Work out the finished part from the listing and answer in its coordinate system (mm). A direction names the side the tool comes from. Round coordinates to 2 decimals unless told otherwise and drop trailing zeros. Loops run counter-clockwise (first coordinate to the right, second up) from the corner with the lowest first, then second, coordinate; pieces in that order, holes last.
from build123d import *

# Parameters (mm, degrees)
ZAOKR_GLENIE2_R  = 2
SFAZOWANIE1_SIZE = 3


with BuildPart() as part:
    # Szkic1 → Obrót1 (revolve)
    with BuildSketch(Plane(origin=(0, 0, 0), x_dir=(1, 0, 0), z_dir=(0, 1, 0))):
        Polygon((15, 65), (-15, 65), (-15, 76), (-7.5, 76), (-7.5, 84), (-15, 84), (-15, 95), (15, 95), (15, 84), (7.5, 84), (7.5, 76), (15, 76), align=None)
    revolve(axis=Axis((0, 0, 0), (-1, 0, 0)))

    # Zaokrąglenie2
    zaokr_glenie2_edges = [part.edges().sort_by_distance(p)[0] for p in [
        (-7.5, 0, 84),
        (7.5, 0, 84),
        (7.5, 0, 76),
    ]]
    fillet(zaokr_glenie2_edges, radius=ZAOKR_GLENIE2_R)

    # Sfazowanie1
    sfazowanie1_edges = [part.edges().sort_by_distance(p)[0] for p in [
        (15, 0, 76),
        (-15, 0, 76),
        (-15, 0, 95),
        (15, 0, 95),
    ]]
    chamfer(sfazowanie1_edges, length=SFAZOWANIE1_SIZE)


solid = part.part
Item 1: Determine the mould class of faces 1 (the face through (7.5, 30, -73)), 2 (the face through (14.854, 89.954, 19.975)), 3 (the face through (15, 43, 49)) for opening direction Y: pulls with the +Y half, pulls with the -Y half, needs draft (parallel to the pull), parting line crosses it, or undercut.
Item 2: Section A-A, the plane x = 1.5 is taken. Give the vertices of the cut face in (y, z), plus the area to 3 significant figures.
Item 3: Straight lines are drawn through the part: line 1 (Y direction, x = -10.85, z = 0); line 2 (Z direction, x = 4.25, y = 0); line 3 (Z direction, x = 13.85, y = 0). For each, find the intervals that lie inside material, in ascending order.
Item 4: Each of these flat-tipped pins is pushed along its axis until it touches: P1, Ø5, axis at x = -1, y = -32, coming from the -Z side; P2, Ø12, axis at x = 6, z = 39, coming from the -Y side; P3, Ø10, axis at x = -5, y = -68, coming from the +Z side. Where does it stop, or does it pass through?
Item 5: For faces 4 (the face through (-9.718, 67.425, -35.069)), 5 (the face through (15, 75, -40)), 6 (the face through (10.768, 67.425, -35.069)), determine the directions among +Z, -Z, +X, -X, +Y, -Y from which every point of the face is accessible in a straight line to the end or side of a thin tool.
Answer below:
1. face 1: undercut
1. face 2: parting line crosses it
1. face 3: needs draft
2. outline: circle Ø190 at (0, 0); hole circle Ø130 at (0, 0)
2. area: 15,100 mm2
3. line 1: y = -95 to -84, -76 to -65, 65 to 76, 84 to 95
3. line 2: z = -95 to -65, 65 to 95
3. line 3: z = -93.15 to -84, -74.15 to -65, 65 to 74.15, 84 to 93.15
4. P1: stops at z = -90.3
4. P2: stops at y = -89.08
4. P3: stops at z = 71.11
5. face 4: -X
5. face 5: +Z, -Z, +X, +Y, -Y
5. face 6: +X
